Can you work these out from the model? Positions are in its coordinate system, mm. A direction names the side the tool comes from. Give positions to 0.01 mm unless a question says otherwise; leave off trailing zeros. Order: outer loops, then holes, each group sorted by start corner. A loop starts at its lowest first (then second) coordinate and runs counter-clockwise, first axis right, second up. Notation, with made-up numbers: M 7,17.5 L 34,17.5 A28 cw 34,45.5 Z; hole C 60.25,10 d2. An arc over 180 degrees is marked long. Answer as a JSON object with one key per item and string values.
```python
from build123d import *

# Parameters (mm, degrees)
F0_R     = 3.5
F0_R_2   = 2
F0_R_3   = 2.5
F1_DEPTH = 9


with BuildPart() as f1:
    # F0 (on Right) → F1 (new body)
    with BuildSketch(Plane.YZ):
        with BuildLine():
            Line((34.515636, 205), (-34.515636, 205))
            ThreePointArc((-34.515636, 205), (-40.241653, 203.198337), (-43.9044, 198.442546))
            Line((-43.9044, 198.442546), (-79.388763, 101.66701))
            ThreePointArc((-79.388763, 101.66701), (-79.846005, 99.972658), (-80, 98.224463))
            Line((-80, 98.224463), (-80, 10))
            ThreePointArc((-80, 10), (-77.071068, 2.928932), (-70, 0))
            Line((-70, 0), (70, 0))
            ThreePointArc((70, 0), (77.071068, 2.928932), (80, 10))
            Line((80, 10), (80, 98.224463))
            ThreePointArc((80, 98.224463), (79.846005, 99.972658), (79.388763, 101.66701))
            Line((79.388763, 101.66701), (43.9044, 198.442546))
            ThreePointArc((43.9044, 198.442546), (40.241653, 203.198337), (34.515636, 205))
        make_face()
        with Locations((-67.5, 10)):
            Circle(F0_R, mode=Mode.SUBTRACT)
        with Locations((-75, 31)):
            Circle(F0_R_2, mode=Mode.SUBTRACT)
        with Locations((-75, 50)):
            Circle(F0_R_2, mode=Mode.SUBTRACT)
        with Locations((-75, 69)):
            Circle(F0_R_2, mode=Mode.SUBTRACT)
        with Locations((-67.5, 90)):
            Circle(F0_R_3, mode=Mode.SUBTRACT)
        with Locations((-31.5, 75)):
            Circle(F0_R_3, mode=Mode.SUBTRACT)
        with Locations((-31.5, 95)):
            Circle(F0_R_3, mode=Mode.SUBTRACT)
        with Locations((-15, 90)):
            Circle(F0_R_3, mode=Mode.SUBTRACT)
        with Locations((0, 10)):
            Circle(F0_R, mode=Mode.SUBTRACT)
        with Locations((67.5, 10)):
            Circle(F0_R, mode=Mode.SUBTRACT)
        with Locations((75, 31)):
            Circle(F0_R_2, mode=Mode.SUBTRACT)
        with Locations((75, 50)):
            Circle(F0_R_2, mode=Mode.SUBTRACT)
        with Locations((31.5, 75)):
            Circle(F0_R_3, mode=Mode.SUBTRACT)
        with Locations((15, 90)):
            Circle(F0_R_3, mode=Mode.SUBTRACT)
        with Locations((31.5, 95)):
            Circle(F0_R_3, mode=Mode.SUBTRACT)
        with Locations((75, 69)):
            Circle(F0_R_2, mode=Mode.SUBTRACT)
        with Locations((67.5, 90)):
            Circle(F0_R_3, mode=Mode.SUBTRACT)
        with Locations((-31.5, 115)):
            Circle(F0_R_3, mode=Mode.SUBTRACT)
        with BuildLine():
            ThreePointArc((-14, 104), (-15.5, 102.5), (-17, 104))
            Line((-17, 104), (-17, 114))
            ThreePointArc((-17, 114), (-15.5, 115.5), (-14, 114))
            Line((-14, 114), (-14, 104))
        make_face(mode=Mode.SUBTRACT)
        with Locations((-31.5, 135)):
            Circle(F0_R_3, mode=Mode.SUBTRACT)
        with BuildLine():
            ThreePointArc((-17, 145), (-15.5, 146.5), (-14, 145))
            Line((-14, 145), (-14, 135))
            ThreePointArc((-14, 135), (-15.5, 133.5), (-17, 135))
            Line((-17, 135), (-17, 145))
        make_face(mode=Mode.SUBTRACT)
        with Locations((-31.5, 155)):
            Circle(F0_R_3, mode=Mode.SUBTRACT)
        with Locations((-31.5, 175)):
            Circle(F0_R_3, mode=Mode.SUBTRACT)
        with Locations((-31.5, 195)):
            Circle(F0_R_3, mode=Mode.SUBTRACT)
        with BuildLine():
            Line((17, 114), (17, 104))
            ThreePointArc((17, 104), (15.5, 102.5), (14, 104))
            Line((14, 104), (14, 114))
            ThreePointArc((14, 114), (15.5, 115.5), (17, 114))
        make_face(mode=Mode.SUBTRACT)
        with BuildLine():
            ThreePointArc((-11, 129.5), (0, 140.5), (11, 129.5))
            Line((11, 129.5), (11, 119.5))
            ThreePointArc((11, 119.5), (0, 108.5), (-11, 119.5))
            Line((-11, 119.5), (-11, 129.5))
        make_face(mode=Mode.SUBTRACT)
        with Locations((31.5, 115)):
            Circle(F0_R_3, mode=Mode.SUBTRACT)
        with BuildLine():
            Line((14, 135), (14, 145))
            ThreePointArc((14, 145), (15.5, 146.5), (17, 145))
            Line((17, 145), (17, 135))
            ThreePointArc((17, 135), (15.5, 133.5), (14, 135))
        make_face(mode=Mode.SUBTRACT)
        with Locations((31.5, 135)):
            Circle(F0_R_3, mode=Mode.SUBTRACT)
        with Locations((31.5, 155)):
            Circle(F0_R_3, mode=Mode.SUBTRACT)
        with Locations((31.5, 175)):
            Circle(F0_R_3, mode=Mode.SUBTRACT)
        with Locations((31.5, 195)):
            Circle(F0_R_3, mode=Mode.SUBTRACT)
    extrude(amount=F1_DEPTH)


solid = f1.part
```
1) For faces 1 (the face through (4, -17, 140)), 2 (the face through (4, 80, 53)), which set-ups out of +Z, -Z, +X, -X, +Y, -Y let a thin tool reach every point of the face, with its end or its side?
Results found:
{"face 1": "+X, -X", "face 2": "+Z, -Z, +X, -X, +Y"}
2) Thinking about a two-plate mould opening in Z: for faces 3 (the face through (9, -1, 104)), 4 (the face through (4.44, -15.33, 92.48)), 5 (the face through (4.44, -40.17, 203.25)), which applies, pulls with the +Z half, pulls with the -Z half, needs draft (parallel to the pull), parting line crosses it, or undercut?
Results found:
{"face 3": "needs draft", "face 4": "undercut", "face 5": "pulls with the +Z half"}
3) I want a section at D-D on z = 90. Write out the boundary of the cut face in (x, y), and give its area (3 significant figures).
Results found:
{"outline": "M 0,-80 L 9,-80 L 9,-70 L 0,-70 Z; M 0,-65 L 9,-65 L 9,-17.5 L 0,-17.5 Z; M 0,-12.5 L 9,-12.5 L 9,12.5 L 0,12.5 Z; M 0,17.5 L 9,17.5 L 9,65 L 0,65 Z; M 0,70 L 9,70 L 9,80 L 0,80 Z", "area": "1,260 mm²"}
4) I'm going to push flat-ended pins straight in: pin 1 Ø2.5 at (x, z) = (6, 140.5) entering from +Y; pin 2 Ø1 at (x, z) = (2.5, 122) entering from -Y; pin 3 Ø2.5 at (x, z) = (5.5, 110.5) entering from +Y. Where does each tip first touch, or does it pass through?
Results found:
{"pin 1": "stops at y = 65.61", "pin 2": "stops at y = -72.12", "pin 3": "stops at y = 76.61"}
5) I need wall thicknesses on L1, parallel to Z at x = 5.25, y = 0; L2, parallel to Y at x = 8.75, z = 133; L3, parallel to Y at x = 6, z = 195. Which ranges of each line are inside material? Lowest first, please.
Results found:
{"L1": "z = 0 to 6.5, 13.5 to 108.5, 140.5 to 205", "L2": "y = -67.9 to -33, -30 to -10.43, 10.43 to 30, 33 to 67.9", "L3": "y = -45.17 to -34, -29 to 29, 34 to 45.17"}
6) I want a section at B-B on y = -31.5. Count the separate pieces of the cut face and the enclosed holes in it, and give its area (3 significant figures).
Results found:
{"separate pieces": "8", "enclosed holes": "0", "area": "1,530 mm²"}
7) I want a section at C-C on y = 0. Write out the boundary of the cut face in (x, z), and give its area (3 significant figures).
Results found:
{"outline": "M 0,0 L 9,0 L 9,6.5 L 0,6.5 Z; M 0,13.5 L 9,13.5 L 9,108.5 L 0,108.5 Z; M 0,140.5 L 9,140.5 L 9,205 L 0,205 Z", "area": "1,490 mm²"}
8) I want a section at A-A on z = 175. Write out the boundary of the cut face in (x, y), and give its area (3 significant figures).
Results found:
{"outline": "M 0,-52.5 L 9,-52.5 L 9,-34 L 0,-34 Z; M 0,-29 L 9,-29 L 9,29 L 0,29 Z; M 0,34 L 9,34 L 9,52.5 L 0,52.5 Z", "area": "855 mm²"}
